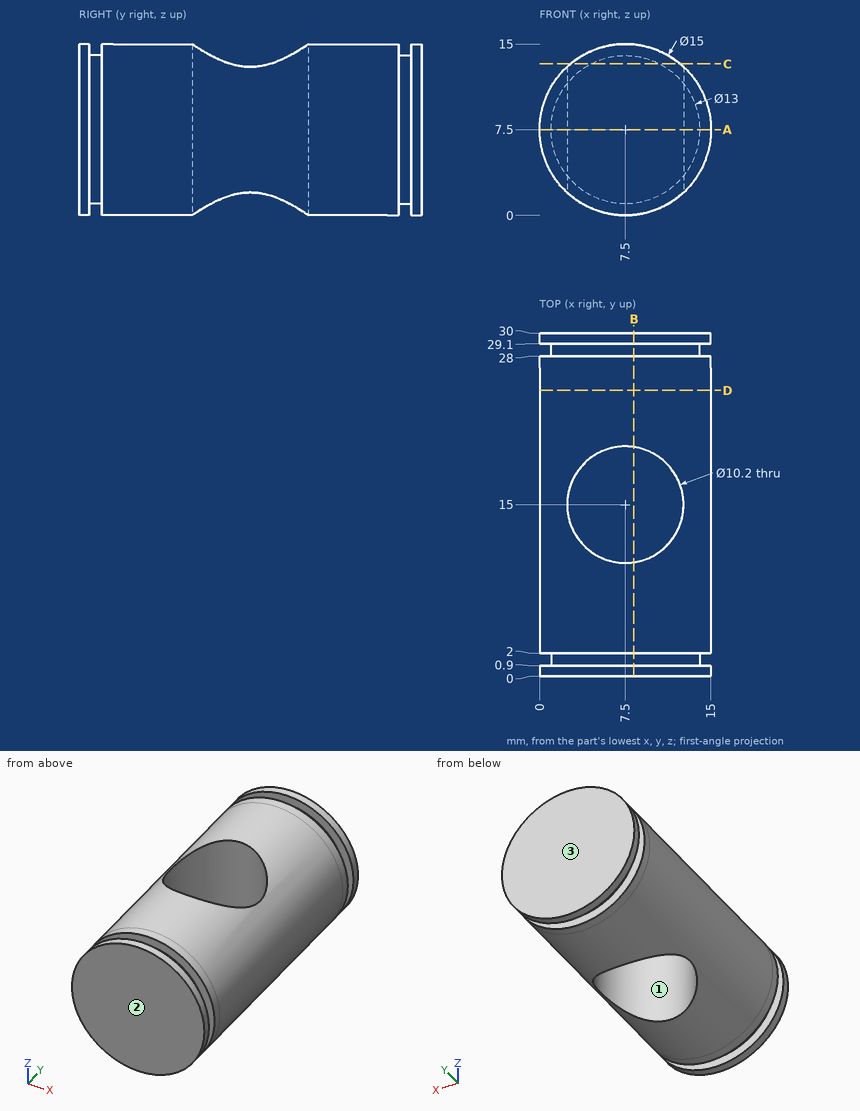
Study the drawing (mm; zero at the part's minimum x, y, z) and answer. Round coordinates to 2 decimals unless told otherwise and drop trailing zeros. Loops run counter-clockwise (first coordinate to the right, second up) from the corner with the lowest first, then second, coordinate; pieces in that order, holes last.
Q1. Section A-A, the plane z = 7.5 is taken. Determine the outline of the cut face in (x, y), then the cut area to 3 significant figures.
Q2. Given pin 1 Ø2 at (x, y) = (11, 15.5) entering from -Z; pin 2 Ø2 at (y, z) = (25.5, 6) entering from -X; pin 3 Ø5 at (x, z) = (9.5, 10) entering from -Y; pin 4 Ø8 at (y, z) = (20.5, 13) entering from +X, each flat-ended and moving along its own axis, determine where each tip first touches the part or whether it passes through.
Q3. Section D-D, the plane y = 25 is taken. Determine the outline of the cut face in (x, z).
Q4. Section B-B, the plane x = 8.25 is taken. Determine the outline of the cut face in (y, z).
Q5. For a pull along Y with two mould halves and no side action, classify the marked faces 1, 2 and 3 as released by +Y, released by -Y, zero draft, split by the parting line, or undercut.
Q6. Find the intervals of material crossed by line 1 (X direction, y = 15, z = 7.5); line 2 (X direction, y = 15, z = 4.5); line 3 (Y direction, x = 3.75, z = 8.5), in increasing order.
Q7. Section C-C, the plane z = 13.25 is taken. Determine the outline of the cut face in (x, y), then the cut area to 3 significant figures.
Completed:
1. outline: (0, 0) - (15, 0) - (15, 0.9) - (14, 0.9) - (14, 2) - (15, 2) - (15, 28) - (14, 28) - (14, 29.1) - (15, 29.1) - (15, 30) - (0, 30) - (0, 29.1) - (1, 29.1) - (1, 28) - (0, 28) - (0, 2) - (1, 2) - (1, 0.9) - (0, 0.9) - close; hole circle Ø10.2 at (7.5, 15)
1. area: 364 mm2
2. pin 1: passes through
2. pin 2: stops at x = 0.02
2. pin 3: stops at y = 0
2. pin 4: stops at x = 14.85
3. outline: circle Ø15 at (7.5, 7.5)
4. outline: (0, 0.04) - (0.9, 0.04) - (0.9, 1.04) - (2, 1.04) - (2, 0.04) - (9.96, 0.04) - (9.96, 14.96) - (2, 14.96) - (2, 13.96) - (0.9, 13.96) - (0.9, 14.96) - (0, 14.96) - close; (20.04, 0.04) - (28, 0.04) - (28, 1.04) - (29.1, 1.04) - (29.1, 0.04) - (30, 0.04) - (30, 14.96) - (29.1, 14.96) - (29.1, 13.96) - (28, 13.96) - (28, 14.96) - (20.04, 14.96) - close
5. face 1: undercut
5. face 2: released by -Y
5. face 3: released by +Y
6. line 1: x = 0 to 2.4, 12.6 to 15
6. line 2: x = 0.63 to 2.4, 12.6 to 14.37
6. line 3: y = 0 to 11.54, 18.46 to 30
7. outline: (2.68, 0) - (12.32, 0) - (12.32, 0.9) - (10.53, 0.9) - (10.53, 2) - (12.32, 2) - (12.32, 13.32) arc R5.1 cw to (2.68, 13.32) - (2.68, 2) - (4.47, 2) - (4.47, 0.9) - (2.68, 0.9) - close; (2.68, 16.68) arc R5.1 cw to (12.32, 16.68) - (12.32, 28) - (10.53, 28) - (10.53, 29.1) - (12.32, 29.1) - (12.32, 30) - (2.68, 30) - (2.68, 29.1) - (4.47, 29.1) - (4.47, 28) - (2.68, 28) - close
7. area: 201 mm2
